```python
from build123d import *

# Parameters (mm, degrees)
F0_R     = 1.5933630383
F1_DEPTH = 3.175
F2_R     = 3.17499


# Not quite as in the source:
# - a fillet or chamfer is up to 0.001 mm smaller than in the source, because OpenCascade refuses the exact size


with BuildPart() as f1:
    # F0 (on Top) → F1 (new body)
    with BuildSketch(Plane.XY):
        Polygon((58.8864982128, 56.2052130699), (-55.4059632123, 56.2052130699), (0, -57.1772865951), align=None)
        with Locations((-5.6359637529, -27.1478164941)):
            Circle(F0_R, mode=Mode.SUBTRACT)
        with Locations((5.7859569788, -27.0903464407)):
            Circle(F0_R, mode=Mode.SUBTRACT)
        with Locations((-41.9265702367, 42.1965457499)):
            Circle(F0_R, mode=Mode.SUBTRACT)
        with Locations((-37.0861701667, 49.9411858618)):
            Circle(F0_R, mode=Mode.SUBTRACT)
        with Locations((43.6793863773, 42.3348434269)):
            Circle(F0_R, mode=Mode.SUBTRACT)
        with Locations((36.7645248771, 49.9411858618)):
            Circle(F0_R, mode=Mode.SUBTRACT)
    extrude(amount=F1_DEPTH)

    # F2 (radius 3.175 in the source; OpenCascade refuses exactly that, so slightly less here)
    f2_edges = [f1.edges().sort_by_distance(p)[0] for p in [
        (-27.702982, -0.486037, 3.175),
        (29.443249, -0.486037, 3.175),
        (1.740268, 56.205213, 3.175),
        (0, -57.177287, 1.5875),
        (-55.405963, 56.205213, 1.5875),
        (58.886498, 56.205213, 1.5875),
    ]]
    fillet(f2_edges, radius=F2_R)


solid = f1.part
```
The listing builds one solid part. Answer for the finished solid, in the listing's coordinates (mm). Coordinates: 2 decimals unless noted, no trailing zeros. Loops run counter-clockwise (first coordinate to the right, second up) from the corner with the lowest first, then second, coordinate; pieces in that order, holes last. Notation, with made-up numbers: M 22.25,14 L 27.25,14 A16 cw 27.25,34 Z; hole C -36.75,-30 d10. An arc over 180 degrees is marked long. Answer as a JSON object with one key per item and string values. Group by question number.
Item 1: Each of these flat-tipped pins is pushed along its axis until it touches: P1, Ø3, axis at x = -37.09, y = 49.94, coming from the -Z side; P2, Ø1.5, axis at y = -24, z = 2, coming from the +X side. Where does it stop, or does it pass through?
Item 2: Consider L1, parallel to Y at x = -6, z = 0.7; L2, parallel to Z at x = -16, y = -18; L3, parallel to Y at x = -36, z = 0.9. Determine where each line is inside the solid, lowest interval first.
Item 3: Section A-A (z = 1.9) is taken. Write down the section's boundary in (x, y), and give its area (3 significant figures).
Item 4: Determine the mould class of faces 1 (the face through (0.94, 55.3, 2.22)), 2 (the face through (35.59, 51.02, 1.57)), 3 (the face through (29.26, 1.13, 2.22)) for opening direction X: +X half, -X half, draft (parallel to the pull), parting line (faces both ways), or undercut.
Solved:
{
 "1": {"P1": "passes through", "P2": "stops at x = 17.1"},
 "2": {"L1": "y = -44.72 to -28.7, -25.6 to 56.13", "L2": "z = 0 to 3.16", "L3": "y = 16.79 to 48.78, 51.11 to 56.07"},
 "3": {"outline": "M -52.61,51.91 L -2.2,-51.24 A2.54 ccw 2.34,-51.29 L 55.92,51.86 A2.54 ccw 53.66,55.57 L -50.32,55.57 A2.54 ccw Z; hole C -41.93,42.2 d3.19; hole C -37.09,49.94 d3.19; hole C -5.64,-27.15 d3.19; hole C 5.79,-27.09 d3.19; hole C 36.76,49.94 d3.19; hole C 43.68,42.33 d3.19", "area": "6,190 mm2"},
 "4": {"face 1": "draft", "face 2": "undercut", "face 3": "+X half"}
}
